from build123d import *

# Parameters (mm, degrees)
F1_DEPTH    = 10
F2_DEPTH    = 6
F3_SIZE2    = 15
F3_SIZE     = 5
F4_T1_DEPTH = 58.6615242271
F5_R        = 13
F6_T1_DEPTH = 18.0508625467


# Not quite as in the source:
# - a fillet or chamfer that OpenCascade refuses, or shapes differently, is made with other operations: its cross-section is extruded or revolved along the edge and cut away or added


with BuildPart() as f1:
    # F0 (on Front) → F1 (new body)
    with BuildSketch(Plane.XZ):
        with BuildLine():
            ThreePointArc((2.15, -0.0081778196), (-3.4744734584, 2.4513486566), (-1.4615047685, -3.3479555451))
            Line((-1.4615047685, -3.3479555451), (-0.9384952315, -3.3479555451))
            ThreePointArc((-0.9384952315, -3.3479555451), (1.2595264762, -2.2826512779), (2.15, -0.0081778196))
        make_face()
    extrude(amount=-F1_DEPTH)

    # F0 (on Front) → F2 (join)
    with BuildSketch(Plane.XZ):
        with BuildLine():
            Line((15.3, 3.3520444549), (-14.7, 3.3520444549))
            Line((-14.7, 3.3520444549), (-14.7, -3.3479555451))
            Line((-14.7, -3.3479555451), (-1.4615047685, -3.3479555451))
            ThreePointArc((-1.4615047685, -3.3479555451), (-3.4744734584, 2.4513486566), (2.15, -0.0081778196))
            ThreePointArc((2.15, -0.0081778196), (1.2595264762, -2.2826512779), (-0.9384952315, -3.3479555451))
            Line((-0.9384952315, -3.3479555451), (15.3, -3.3479555451))
            Line((15.3, -3.3479555451), (15.3, 3.3520444549))
        make_face()
        with BuildLine():
            ThreePointArc((2.15, -0.0081778196), (-3.4744734584, 2.4513486566), (-1.4615047685, -3.3479555451))
            Line((-1.4615047685, -3.3479555451), (-0.9384952315, -3.3479555451))
            ThreePointArc((-0.9384952315, -3.3479555451), (1.2595264762, -2.2826512779), (2.15, -0.0081778196))
        make_face()
    extrude(amount=F2_DEPTH)

    # F3
    f3_edges = [f1.edges().sort_by_distance(p)[0] for p in [
        (15.3, -6, 0.002044),
    ]]
    f3_side = f1.faces().sort_by_distance((15.3, -3, 0.002044))[0]
    chamfer(f3_edges, length=F3_SIZE, length2=F3_SIZE2, reference=f3_side)

    # F4: fillet of radius 12 on 1 edges, made by hand

    # F4_s2 → F4_t1 (cut)
    with BuildSketch(Plane.XY.offset(-29.3287176586)):
        with BuildLine():
            ThreePointArc((-4.3076951546, -6), (-10.3076951546, -4.3923048454), (-14.7, 0))
            Line((-14.7, 0), (-14.7, -6))
            Line((-14.7, -6), (-4.3076951546, -6))
        make_face()
    extrude(amount=F4_T1_DEPTH, mode=Mode.SUBTRACT)

    # F5
    f5_edges = [f1.edges().sort_by_distance(p)[0] for p in [
        (0.3, -6, 0.002044),
    ]]
    fillet(f5_edges, radius=F5_R)

    # F6: fillet of radius 4 on 1 edges, made by hand

    # F6_s2 → F6_t1 (cut)
    with BuildSketch(Plane.XY.offset(-9.0233868185)):
        with BuildLine():
            ThreePointArc((13.1463252567, -1.7178915811), (14.3757224349, -1.0502059409), (15.3, 0))
            Line((15.3, 0), (15.3, -1))
            Line((15.3, -1), (13.1463252567, -1.7178915811))
        make_face()
    extrude(amount=F6_T1_DEPTH, mode=Mode.SUBTRACT)


solid = f1.part
Build history of the part. All positions in model axes, mm. Round coordinates to 2 decimals unless told otherwise and drop trailing zeros. Write each loop counter-clockwise with the first axis right and the second up, starting at its lowest first coordinate (ties: lowest second). Pieces come first, ordered by that corner, then holes. Notation, with made-up numbers: (-10.5, 48) -> (26.5, 48) arc R11 ccw to (26.5, 68) -> close; hole circle Ø3 at (32, 30). An arc over 180 degrees is marked (long way). Write item = value, one per line.
(1) Band-saw the part on B-B (x = 1). Give the cut face in (y, z), then the cut area to 3 significant figures.
Answer:
outline = (-5.69, -3.35) -> (0, -3.35) -> (0, -2.53) -> (10, -2.53) -> (10, 2.52) -> (0, 2.52) -> (0, 3.35) -> (-5.69, 3.35) -> close
area = 88.7 mm2
(2) Flat gauge pins, fed straight in: pin 1 (3 mm diameter, centred on x = 6, z = 2.5, fed in from -Y); pin 2 (1 mm diameter, centred on y = -2.5, z = 2.5, fed in from -X); pin 3 (2 mm diameter, centred on y = -1.5, z = 2.5, fed in from +X). Where does each tip first touch, or does it go through?
Answer:
pin_1 = -4.6
pin_2 = -13.25
pin_3 = 14.94
(3) Band-saw the part on A-A (z = -1). Give the cut face in (x, y), then the cut area to 3 significant figures.
Answer:
outline = (-14.7, 0) arc R12 ccw to (-4.31, -6) -> (-1.81, -6) arc R13 ccw to (2.3, -5.33) -> (13.15, -1.72) arc R4 ccw to (15.3, 0) -> (2, 0) -> (2, 10) -> (-4.4, 10) -> (-4.4, 0) -> close
area = 188 mm2
(4) Probe L1, parallel to Y at x = -1.5, z = 2; L2, parallel to X at y = 6.75, z = -0.25; L3, parallel to X at y = 5.5, z = 2. List the from-to ranges inside material, lowest first.
Answer:
L1 = -6 to 10
L2 = -4.54 to 2.14
L3 = -3.88 to 1.48
(5) Band-saw the part on D-D (y = -1.25). Give the cut face in (x, z), then the cut area to 3 significant figures.
Answer:
outline = (-13.87, -3.35) -> (14.1, -3.35) -> (14.1, 3.35) -> (-13.87, 3.35) -> close
area = 187 mm2
(6) Band-saw the part on C-C (y = 3). Give the cut face in (x, z).
Answer:
outline = (-1.46, -3.35) -> (-0.94, -3.35) arc R3.35 ccw (long way) to start
